Input: part model. Units: mm. Frame: model coordinates. Face numbers are marked on the shaded views. A direction names the side the tool comes from. Give positions to 0.01 mm unless a question says otherwise; leave off trailing zeros. Loops run counter-clockwise (first coordinate to the right, second up) from the corner with the lowest first, then second, coordinate; pieces in that order, holes last. Notation, with made-up numbers: (86.5, 85.25) -> (109.5, 85.25) arc R10 ccw to (109.5, 93.25) -> close; hole circle Ø7 at (64, 48.25). An arc over 180 degrees is marked (long way). Use CSV: the item, a comma, the result in double quotes.
Autodesk Inventor part; units mm, degrees
ref_plane "YZ Plane" through (0, 0, 0) normal (1, 0, 0) x (0, 1, 0)
ref_plane "XZ Plane" through (0, 0, 0) normal (0, 1, 0) x (-1, 0, 0)
ref_plane "XY Plane" through (0, 0, 0) normal (0, 0, 1) x (1, 0, 0)
sketch "Sketch1" plane through (0, 0, 0) normal (0, 1, 0) x (-1, 0, 0)
  line L0 (2.1, 1.5) -> (-2.1, 1.5)
  line L1 (-2.1, -1.5) -> (2.1, -1.5)
  line L2 (7, 0) -> (-7, 0) construction
  line L3 (0, -5.6) -> (0, 5.6) construction
  line L4 (5, 4) -> (-5, 4)
  line L5 (-5, 4) -> (-5, -4)
  line L6 (-5, -4) -> (5, -4)
  line L7 (5, -4) -> (5, 4)
  line L8 (-2, 0.84) -> (-2, -0.76)
  line L9 (2, -0.76) -> (2, 0.84)
  line L10 (-2.1, 1.5) -> (-2.1, -1.5)
  line L11 (2.1, -1.5) -> (2.1, 1.5)
  line L12 (0.2, 1.5) -> (-0.2, 1.5)
  point P0 (0, 0)
  point P1 (2.3, 0)
  point P2 (0, 1.5)
  dimension "d2" = 3
  dimension "d3" = 10
  dimension "d16" = 2.5
  dimension "d17" = 2.5
  dimension "d29" = 0.1
  dimension "d30" = 0.1
extrude "Extrusion1" add sketch "Sketch1" along normal blind 4
sketch "Sketch2" plane through (-5, 0, 4) normal (0, 0, 1) x (1, 0, 0)
  circle A0 centre (5, 1.8) radius 1.5
  line L0 (0, 4) -> (10, 4) construction
  line L1 (5, -1.76) -> (5, 10.56) construction
  line L2 (0, 0) -> (0, 4)
  arc A1 (7, 8.5082) -> (3, 8.5082) centre (5, 1.8) ccw
  point P0 (5, 0)
  point P1 (0, 2)
  dimension "d7" = 3
extrude "Extrusion2" add sketch "Sketch2" along normal blind 5
sketch "Sketch4" plane through (5, 0, -4) normal (0, 0, -1) x (-1, 0, 0)
  circle A0 centre (5, 1.8) radius 0.2 construction
  circle A1 centre (5, 1.8) radius 0.5
  line L0 (4.6464, 2.1536) -> (5, 2.5071)
  line L1 (5, 2.5071) -> (5.3536, 2.1536)
  point P0 (5, 0)
  dimension "d18" = 1
extrude "Extrusion4" cut sketch "Sketch4" against normal blind 1
chamfer "Chamfer2" distance 0.2 angle 45 3 edges at (-0.1768, 2.3303, -4) (0, 1.3, -4) (0.1768, 2.3303, -4)
chamfer "Chamfer3" distance 0.5 angle 45 1 edges at (-1.5, 1.8, 9)
fillet "Fillet1" radius 0.5 1 edges at (-1.5, 1.8, 4)
fillet "Fillet2" radius 1 4 edges at (-5, 2, 4) (-5, 2, -4) (5, 2, -4) (5, 2, 4)
properties part number "Pen_nib_stopper"
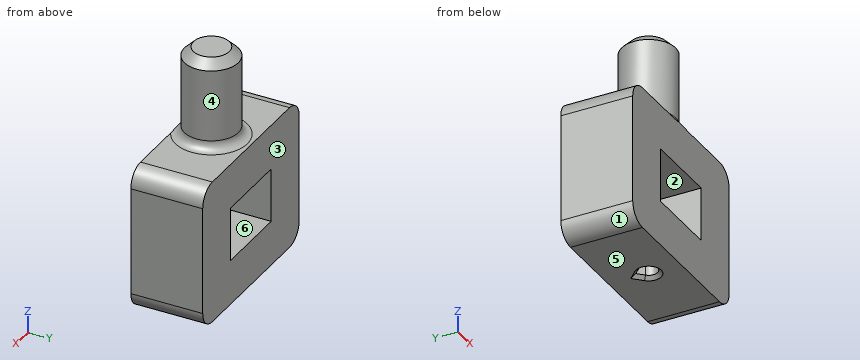
1) Section query A-A (z = 1). Return loops of the section in (x, y), then the cut area to 3 significant figures.
From the geometry:
outline,"(-5, 0) -> (-2.1, 0) -> (-2.1, 4) -> (-5, 4) -> close; (2.1, 0) -> (5, 0) -> (5, 4) -> (2.1, 4) -> close"
area,"23.2 mm^2"
2) Section query B-B (y = 1.8). Return loops of the section in (x, z).
From the geometry:
outline,"(-5, -3) arc R1 ccw to (-4, -4) -> (-0.7, -4) -> (-0.5, -3.8) -> (-0.5, -3) -> (0.5, -3) -> (0.5, -3.8) -> (0.7, -4) -> (4, -4) arc R1 ccw to (5, -3) -> (5, 3) arc R1 ccw to (4, 4) -> (2, 4) arc R0.5 cw to (1.5, 4.5) -> (1.5, 8.5) -> (1, 9) -> (-1, 9) -> (-1.5, 8.5) -> (-1.5, 4.5) arc R0.5 cw to (-2, 4) -> (-4, 4) arc R1 ccw to (-5, 3) -> close; hole (-2.1, -1.5) -> (2.1, -1.5) -> (2.1, 1.5) -> (-2.1, 1.5) -> close"
3) Ray query, line 1 (X direction, y = 3.15, z = 1); line 2 (Z direction, x = 3, y = 0.5); line 3 (Z direction, x = -1, y = 0.2). Return the intervals inside material, ascending.
From the geometry:
line 1,"x = -5 to -2.1, 2.1 to 5"
line 2,"z = -4 to 4"
line 3,"z = -4 to -1.5, 1.5 to 4.01"
4) Reachability of the marked faces 4, 5 and 6 from +Z, -Z, +X, -X, +Y, -Y: full face, straight path, thin tool, end or side. Return the list, or none.
From the geometry:
face 4,"+Z"
face 5,"-Z, +X, -X, +Y, -Y"
face 6,"+Y, -Y"
5) Mould query, pull axis Z, two halves, no side actions, for the marked faces 1, 2 and 3. Classes: pulls with the +Z half, pulls with the -Z half, needs draft (parallel to the pull), parting line crosses it, or undercut.
From the geometry:
face 1,"pulls with the -Z half"
face 2,"undercut"
face 3,"needs draft"
6) Section query C-C (x = -2.25). Return loops of the section in (y, z).
From the geometry:
outline,"(0, -4) -> (4, -4) -> (4, 4) -> (0, 4) -> close"
